Source: CAD feature listing. Evaluate the final solid. Frame: model axes, mm. A direction names the side the tool comes from. Round coordinates to 2 decimals unless told otherwise and drop trailing zeros. Write each loop counter-clockwise with the first axis right and the second up, starting at its lowest first coordinate (ties: lowest second). Pieces come first, ordered by that corner, then holes.
from build123d import *

# Parameters (mm, degrees)
CYLINDER_R        = 1.7
CYLINDER_DEPTH    = 10
CYLINDER001_R     = 1.7
CYLINDER001_DEPTH = 10
BOX_W             = 50
BOX_H             = 6
BOX_DEPTH         = 5
CHAMFER_1_SIZE2   = 2.9
CHAMFER_1_SIZE    = 4.9
CHAMFER_2_SIZE2   = 2.9
CHAMFER_2_SIZE    = 4.9
BOX001_W          = 50
BOX001_H          = 20
BOX001_DEPTH      = 5
CHAMFER001_SIZE   = 2
FILLET_R          = 0.3


with BuildPart() as cylinder:
    # Cylinder → Cylinder (new body)
    with BuildSketch(Plane(origin=(10, 15, 0), x_dir=(1, 0, 0), z_dir=(0, 0, 1))):
        Circle(CYLINDER_R)
    extrude(amount=CYLINDER_DEPTH)


with BuildPart() as cylinder001:
    # Cylinder001 → Cylinder001 (new body)
    with BuildSketch(Plane(origin=(40, 15, 0), x_dir=(1, 0, 0), z_dir=(0, 0, 1))):
        Circle(CYLINDER001_R)
    extrude(amount=CYLINDER001_DEPTH)


with BuildPart() as chamfer_body:
    # Box → Box (new body)
    with BuildSketch(Plane.XY.offset(2)):
        with Locations((25, 3)):
            Rectangle(BOX_W, BOX_H)
    extrude(amount=BOX_DEPTH)

    # Chamfer 1
    chamfer_1_edges = [chamfer_body.edges().sort_by_distance(p)[0] for p in [
        (25, 6, 2),
    ]]
    chamfer_1_side = chamfer_body.faces().sort_by_distance((25, 6, 4.5))[0]
    chamfer(chamfer_1_edges, length=CHAMFER_1_SIZE, length2=CHAMFER_1_SIZE2, reference=chamfer_1_side)

    # Chamfer 2
    chamfer_2_edges = [chamfer_body.edges().sort_by_distance(p)[0] for p in [
        (25, 0, 2),
    ]]
    chamfer_2_side = chamfer_body.faces().sort_by_distance((25, 0, 4.5))[0]
    chamfer(chamfer_2_edges, length=CHAMFER_2_SIZE, length2=CHAMFER_2_SIZE2, reference=chamfer_2_side)


with BuildPart() as chamfer_body_1:
    # Chamfer placement: moved
    add(chamfer_body.part.moved(Location((0, 3, 0))))


with BuildPart() as fillet_body:
    # Box001 → Box001 (new body)
    with BuildSketch(Plane.XY):
        with Locations((25, 10)):
            Rectangle(BOX001_W, BOX001_H)
    extrude(amount=BOX001_DEPTH)

    # Cut: cut Chamfer body
    add(chamfer_body_1.part, mode=Mode.SUBTRACT)

    # Cut001: cut Cylinder001
    add(cylinder001.part, mode=Mode.SUBTRACT)

    # Cut002: cut Cylinder
    add(cylinder.part, mode=Mode.SUBTRACT)

    # Chamfer001
    chamfer001_edges = [fillet_body.edges().sort_by_distance(p)[0] for p in [
        (8.3, 15, 5),
        (38.3, 15, 5),
    ]]
    chamfer(chamfer001_edges, length=CHAMFER001_SIZE)

    # Fillet
    fillet_edges = [fillet_body.edges().sort_by_distance(p)[0] for p in [
        (0, 13.937755, 5),
        (25, 7.87551, 5),
        (50, 13.937755, 5),
        (25, 20, 5),
        (0, 2.062245, 5),
        (0, 5.012245, 3.5),
        (0, 6.987755, 3.5),
        (0, 20, 2.5),
        (0, 10, 0),
        (0, 0, 2.5),
        (50, 6.987755, 3.5),
        (25, 20, 0),
        (50, 20, 2.5),
        (50, 2.062245, 5),
        (50, 5.012245, 3.5),
        (50, 10, 0),
        (50, 0, 2.5),
        (8.3, 15, 0),
        (25, 4.12449, 5),
        (25, 0, 5),
        (25, 0, 0),
        (38.3, 15, 0),
    ]]
    fillet(fillet_edges, radius=FILLET_R)


solid = fillet_body.part
1) Section query B-B on z = 0.75. Return the cut outline in (x, y).
Taken from the geometry:
outline: (0, 0.3) arc R0.3 ccw to (0.3, 0) - (49.7, 0) arc R0.3 ccw to (50, 0.3) - (50, 19.7) arc R0.3 ccw to (49.7, 20) - (0.3, 20) arc R0.3 ccw to (0, 19.7) - close; hole circle Ø3.4 at (10, 15); hole circle Ø3.4 at (40, 15)
2) Section query A-A on x = 40. Return the cut outline in (y, z), then the cut area to 3 significant figures.
Taken from the geometry:
outline: (0, 0.3) arc R0.3 ccw to (0.3, 0) - (13, 0) arc R0.3 ccw to (13.3, 0.3) - (13.3, 3) - (11.3, 5) - (8.05, 5) arc R0.3 ccw to (7.79, 4.85) - (6.1, 2) - (5.9, 2) - (4.21, 4.85) arc R0.3 ccw to (3.95, 5) - (0.3, 5) arc R0.3 ccw to (0, 4.7) - close; (16.7, 0.3) arc R0.3 ccw to (17, 0) - (19.7, 0) arc R0.3 ccw to (20, 0.3) - (20, 4.7) arc R0.3 ccw to (19.7, 5) - (18.7, 5) - (16.7, 3) - close
area: 72.9 mm2
3) Section query C-C on y = 15. Return the cut outline in (x, z), then the cut area to 3 significant figures.
Taken from the geometry:
outline: (0, 0.3) arc R0.3 ccw to (0.3, 0) - (8, 0) arc R0.3 ccw to (8.3, 0.3) - (8.3, 3) - (6.3, 5) - (0.3, 5) arc R0.3 ccw to (0, 4.7) - close; (11.7, 0.3) arc R0.3 ccw to (12, 0) - (38, 0) arc R0.3 ccw to (38.3, 0.3) - (38.3, 3) - (36.3, 5) - (13.7, 5) - (11.7, 3) - close; (41.7, 0.3) arc R0.3 ccw to (42, 0) - (49.7, 0) arc R0.3 ccw to (50, 0.3) - (50, 4.7) arc R0.3 ccw to (49.7, 5) - (43.7, 5) - (41.7, 3) - close
area: 208 mm2
4) Material intervals for line 1 (Y direction, x = 10, z = 1.9); line 2 (X direction, y = 15, z = 0.95); line 3 (Y direction, x = 11, z = 2.9), sorted ascending.
Taken from the geometry:
line 1: y = 0 to 13.3, 16.7 to 20
line 2: x = 0 to 8.3, 11.7 to 38.3, 41.7 to 50
line 3: y = 0 to 5.37, 6.63 to 13.63, 16.37 to 20
5) Section query D-D on x = 26. Return the cut outline in (y, z).
Taken from the geometry:
outline: (0, 0.3) arc R0.3 ccw to (0.3, 0) - (19.7, 0) arc R0.3 ccw to (20, 0.3) - (20, 4.7) arc R0.3 ccw to (19.7, 5) - (8.05, 5) arc R0.3 ccw to (7.79, 4.85) - (6.1, 2) - (5.9, 2) - (4.21, 4.85) arc R0.3 ccw to (3.95, 5) - (0.3, 5) arc R0.3 ccw to (0, 4.7) - close
6) Pull-direction query (X, two-part tool) for faces 1 (the face through (49.914, 4.99, 3.36)), 2 (the face through (38.65, 13.97, 1.63)), 3 (the face through (0.086, 4.99, 3.36)); classes: released by +X, released by -X, zero draft, split by the parting line, or undercut.
Taken from the geometry:
face 1: released by +X
face 2: undercut
face 3: released by -X
7) Reachability of faces 4 (the face through (49.91, 7.006, 3.363)), 5 (the face through (0.086, 7.01, 3.36)), 6 (the face through (24.654, 5.068, 3.406)), 7 (the face through (0, 10, 2)) from +Z, -Z, +X, -X, +Y, -Y: full face, straight path, thin tool, end or side. Return the list, or none.
Taken from the geometry:
face 4: +Z, +X
face 5: +Z, -X
face 6: +Z, +X, -X
face 7: +Z, -Z, -X, +Y, -Y
